Part model, mm, in its own coordinate system. A direction names the side the tool comes from. Round coordinates to 2 decimals unless told otherwise and drop trailing zeros. Loops run counter-clockwise (first coordinate to the right, second up) from the corner with the lowest first, then second, coordinate; pieces in that order, holes last. Notation, with made-up numbers: M 17,-21 L 23,-21 A10 ccw 23,-13 Z; hole C 61.25,67 d10. An arc over 180 degrees is marked long. Answer as CSV lines item,"result". Start each with the question number.
Item 1: Band-saw the part on C-C (y = 8.5). Give the cut face in (x, z).
Item 2: Wall check: line 1 (Y direction, x = 21.5, z = 14.5); line 2 (Z direction, x = 13.5, y = 8); line 3 (X direction, y = 14.5, z = 24.25). Give the ranges that are in metal, low to high.
Item 3: Mould opens along Y. For faces 1 (the flat face through (20, 0, 13)), 2 (the flat face through (0, 17, 13)), 3 (the flat face through (26, 18, 5.08)) say: pulls with the +Y half, pulls with the -Y half, needs draft (parallel to the pull), parting line crosses it, or undercut.
Item 4: Band-saw the part on A-A (z = 22). Give the cut face in (x, y), and give its area (3 significant figures).
Item 5: Which spindle directions (+Z, -Z, +X, -X, +Y, -Y) get a long thin tool onto all of the face, cutting with end or side? Do faces 4 (the flat face through (20, 17, 0)), 5 (the flat face through (24, 29.095, 15)). Say none if no direction does.
Item 6: Drop flat-ended pins along their axis: pin 1 Ø1.5 at (x, y) = (11, 16) entering from +Z; pin 2 Ø7.5 at (y, z) = (16, 20.5) entering from +X; pin 3 Ø6.5 at (x, y) = (25.5, 22.5) entering from +Z. Give the stop position or say it passes through.
Item 7: Band-saw the part on B-B (x = 22.5). Give the cut face in (y, z).
```python
from build123d import *

# Parameters (mm, degrees)
F0_W     = 40.996857
F0_H     = 34.384463
F1_DEPTH = 25.4
F2_W     = 34.38446
F2_H     = 22.48215
F3_DEPTH = 20.32
F4_R     = 5.08


with BuildPart() as f1:
    # F0 (on Top) → F1 (new body)
    with BuildSketch(Plane.XY):
        with Locations((20.498428, 17.192231)):
            Rectangle(F0_W, F0_H)
    extrude(amount=F1_DEPTH)

    # F2 (on face) → F3 (cut)
    with BuildSketch(Plane.XY.offset(25.4)):
        with Locations((23.804627, 17.853472)):
            Rectangle(F2_W, F2_H)
    extrude(amount=-F3_DEPTH, mode=Mode.SUBTRACT)

    # F4
    f4_edges = [f1.edges().sort_by_distance(p)[0] for p in [
        (6.612397, 17.853472, 5.08),
    ]]
    fillet(f4_edges, radius=F4_R)


solid = f1.part
```
Answer block:
1,outline,"M 0,0 L 41,0 L 41,5.08 L 11.69,5.08 A5.08 cw 6.61,10.16 L 6.61,25.4 L 0,25.4 Z"
2,line 1,"y = 0 to 6.61, 29.09 to 34.38"
2,line 2,"z = 0 to 5.08"
2,line 3,"x = 0 to 6.61"
3,face 1,"pulls with the -Y half"
3,face 2,"needs draft"
3,face 3,"undercut"
4,outline,"M 0,0 L 41,0 L 41,6.61 L 6.61,6.61 L 6.61,29.09 L 41,29.09 L 41,34.38 L 0,34.38 Z"
4,area,"637 mm^2"
5,face 4,"-Z, +X, -X, +Y, -Y"
5,face 5,"+Z, +X"
6,pin 1,"stops at z = 5.29"
6,pin 2,"stops at x = 6.61"
6,pin 3,"stops at z = 5.08"
7,outline,"M 0,0 L 34.38,0 L 34.38,25.4 L 29.09,25.4 L 29.09,5.08 L 6.61,5.08 L 6.61,25.4 L 0,25.4 Z"
